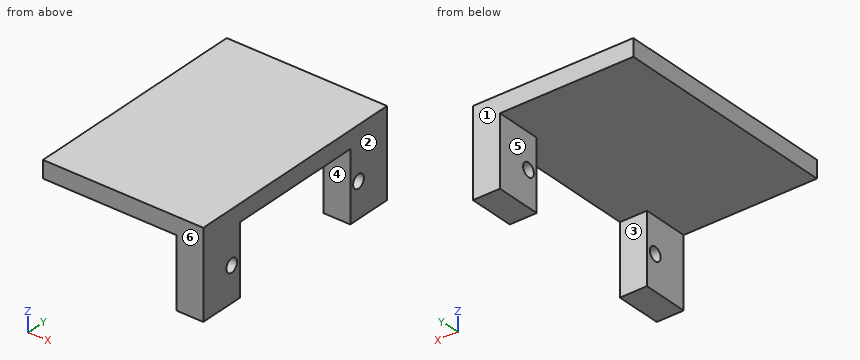
```python
from build123d import *

# Parameters (mm, degrees)
BOSS_EXTRUDE1_DEPTH = 40
SKETCH2_W           = 12.1
SKETCH2_H           = 24
CUT_EXTRUDE3_DEPTH  = 4.7
SKETCH4_R           = 1.175
CUT_EXTRUDE4_DEPTH  = 4.7


with BuildPart() as part:
    # Sketch1 → Boss-Extrude1 (new body)
    with BuildSketch(Plane(origin=(0, 0, 0), x_dir=(1, 0, 0), z_dir=(0, 1, 0))):
        Polygon((0, 12.1), (4.7, 12.1), (4.7, -3), (-23.2, -3), (-23.2, 0), (0, 0), align=None)
    extrude(amount=BOSS_EXTRUDE1_DEPTH)

    # Sketch2 → Cut-Extrude3 (cut)
    with BuildSketch(Plane(origin=(4.7, 0, 0), x_dir=(0, 0, -1), z_dir=(1, 0, 0))):
        with Locations((6.05, 20)):
            Rectangle(SKETCH2_W, SKETCH2_H)
    extrude(amount=-CUT_EXTRUDE3_DEPTH, mode=Mode.SUBTRACT)

    # Sketch4 → Cut-Extrude4 (cut)
    with BuildSketch(Plane(origin=(4.7, 0, 0), x_dir=(0, 0, -1), z_dir=(1, 0, 0))):
        with Locations((6.05, 33.8)):
            Circle(SKETCH4_R)
        with Locations((6.05, 6.2)):
            Circle(SKETCH4_R)
    extrude(amount=-CUT_EXTRUDE4_DEPTH, mode=Mode.SUBTRACT)


solid = part.part
```
Design review of the part built by this model. Coordinates are the model's own, in mm. Face numbers are marked on the shaded views. A direction names the side the tool comes from. Round coordinates to 2 decimals unless told otherwise and drop trailing zeros. Order: outer loops, then holes, each group sorted by start corner. A loop starts at its lowest first (then second) coordinate and runs counter-clockwise, first axis right, second up. Notation, with made-up numbers: M 12.25,46.25 L 59.25,46.25 A13 cw 59.25,68.25 Z; hole C 18,17.25 d1. An arc over 180 degrees is marked long. Put each result on its own line as item: value.
Q1. Consider section D-D (x = -6.5). State the section outline as (y, z) points.
Reported:
outline: M 0,0 L 40,0 L 40,3 L 0,3 Z
Q2. To check wall thickness, follow line 1 (Y direction, x = 1.65, z = -6.05) (3 decimals); line 2 (Z direction, x = -3.25, y = 22.5); line 3 (X direction, y = 3.5, z = -6.25). State the ranges of each line that lie inside material, in increasing order.
Reported:
line 1: 0 to 5.025, 7.375 to 8, 32 to 32.625, 34.975 to 40
line 2: 0 to 3
line 3: 0 to 4.7
Q3. Insertion check: pin 1 Ø9 at (y, z) = (3, -6) entering from -X; pin 2 Ø2 at (x, y) = (-1.5, 14) entering from -Z; pin 3 Ø8 at (x, z) = (0.5, -2.5) entering from -Y. Each pin has a flat end and moves straight along its axis. Give the tip position at first contact, or say it passes through.
Reported:
pin 1: x = 0
pin 2: z = 0
pin 3: y = 0
Q4. Consider section A-A (z = -6.05). State the section outline as (x, y) points (3 decimals), and give its area (3 significant figures).
Reported:
outline: M 0,0 L 4.7,0 L 4.7,5.025 L 0,5.025 Z; M 0,7.375 L 4.7,7.375 L 4.7,8 L 0,8 Z; M 0,32 L 4.7,32 L 4.7,32.625 L 0,32.625 Z; M 0,34.975 L 4.7,34.975 L 4.7,40 L 0,40 Z
area: 53.1 mm²
Q5. Draft analysis for pull direction Y (two halves, no side actions). For the marked faces 1, 2 and 3, state which applies: released by +Y, released by -Y, zero draft, split by the parting line, or undercut.
Reported:
face 1: released by +Y
face 2: zero draft
face 3: undercut
Q6. Machinability: for the marked faces 4, 5 and 6, which of the approach directions +Z, -Z, +X, -X, +Y, -Y give a long, thin tool a straight path to every point of the face, cutting with its end or side? Answer none if there is none.
Reported:
face 4: -Z, +X, -X
face 5: -Z, -X, +Y, -Y
face 6: +Z, -Z, +X, -X, -Y
Q7. Consider section B-B (y = 33.8). State the section outline as (x, z) points (3 decimals).
Reported:
outline: M -23.2,0 L 0,0 L 0,-4.875 L 4.7,-4.875 L 4.7,3 L -23.2,3 Z; M 0,-12.1 L 4.7,-12.1 L 4.7,-7.225 L 0,-7.225 Z
Q8. Consider section C-C (z = -2). State the section outline as (x, y) points, and give its area (3 significant figures).
Reported:
outline: M 0,0 L 4.7,0 L 4.7,8 L 0,8 Z; M 0,32 L 4.7,32 L 4.7,40 L 0,40 Z
area: 75.2 mm²
